```python
from build123d import *

# Parameters (mm, degrees)
F0_W         = 50.8
F0_H         = 50.8
F1_DEPTH     = 50.8
F2_R         = 2.2225
F3_DEPTH     = 3.175
F5_R         = 5.08
F6_T1_DEPTH  = 40.64
F6_T3_DEPTH  = 58.42
F6_T6_ANGLE  = 90
F6_T10_DEPTH = 26.67
F6_T16_DEPTH = 26.67
F6_T22_DEPTH = 26.67
F6_T27_ANGLE = 90
F6_T31_DEPTH = 26.67
F6_T38_DEPTH = 26.67
F6_T44_DEPTH = 26.67
F6_T48_ANGLE = 90
F6_T50_ANGLE = 90
F7_R         = 3.175
F8_DEPTH     = 15.24
F7_W         = 1.27
F7_H         = 6.35
F9_DEPTH     = 8.255


# Not quite as in the source:
# - a fillet or chamfer that OpenCascade refuses, or shapes differently, is made with other operations: its cross-section is extruded or revolved along the edge and cut away or added
# - a feature of the source that left no trace in its solid (it failed there, or was rolled back) is left out


with BuildPart() as f1:
    # F0 (on Top) → F1 (new body)
    with BuildSketch(Plane.XY):
        with Locations((-4.6946440548, -2.4632510453)):
            Rectangle(F0_W, F0_H)
    extrude(amount=F1_DEPTH)

    # F2 (on face) → F3 (join)
    with BuildSketch(Plane(origin=(0, 22.9367489547, 0), x_dir=(-1, 0, 0), z_dir=(0, 1, 0))):
        Polygon((-0.3853559452, 62.23), (-0.3853559452, 53.34), (9.7746440548, 53.34), (9.7746440548, 62.23), (8.5046440548, 63.5), (0.8846440548, 63.5), align=None)
        with Locations((4.6946440548, 58.42)):
            Circle(F2_R, mode=Mode.SUBTRACT)
        Polygon((-0.3853559452, 53.34), (-1.6553559452, 50.8), (11.0446440548, 50.8), (9.7746440548, 53.34), align=None)
    extrude(amount=-F3_DEPTH)

    # F5
    f5_edges = [f1.edges().sort_by_distance(p)[0] for p in [
        (-30.094644, -2.463251, 50.8),
        (20.705356, -2.463251, 50.8),
    ]]
    fillet(f5_edges, radius=F5_R)

    # F6: fillet of radius 5.08 on 11 edges, made by hand

    # F6_s2 → F6_t1 (cut)
    with BuildSketch(Plane.YZ.offset(-25.0146440548)):
        with BuildLine():
            ThreePointArc((-27.8632510453, 45.72), (-26.3753534938, 49.3121024484), (-22.7832510453, 50.8))
            Line((-22.7832510453, 50.8), (-27.8632510453, 50.8))
            Line((-27.8632510453, 50.8), (-27.8632510453, 45.72))
        make_face()
    extrude(amount=F6_T1_DEPTH, mode=Mode.SUBTRACT)

    # F6_s4 → F6_t3 (cut)
    with BuildSketch(Plane.XY.offset(-12.7)):
        with BuildLine():
            ThreePointArc((-30.0946440548, 17.8567489547), (-28.6067465032, 21.4488514031), (-25.0146440548, 22.9367489547))
            Line((-25.0146440548, 22.9367489547), (-30.0946440548, 22.9367489547))
            Line((-30.0946440548, 22.9367489547), (-30.0946440548, 17.8567489547))
        make_face()
        with BuildLine():
            ThreePointArc((-30.0946440548, -22.7832510453), (-28.6067465032, -26.3753534938), (-25.0146440548, -27.8632510453))
            Line((-25.0146440548, -27.8632510453), (-30.0946440548, -27.8632510453))
            Line((-30.0946440548, -27.8632510453), (-30.0946440548, -22.7832510453))
        make_face()
        with BuildLine():
            ThreePointArc((15.6253559452, 22.9367489547), (19.2174583937, 21.4488514031), (20.7053559452, 17.8567489547))
            Line((20.7053559452, 17.8567489547), (20.7053559452, 22.9367489547))
            Line((20.7053559452, 22.9367489547), (15.6253559452, 22.9367489547))
        make_face()
        with BuildLine():
            ThreePointArc((15.6253559452, -27.8632510453), (19.2174583937, -26.3753534938), (20.7053559452, -22.7832510453))
            Line((20.7053559452, -22.7832510453), (20.7053559452, -27.8632510453))
            Line((20.7053559452, -27.8632510453), (15.6253559452, -27.8632510453))
        make_face()
    extrude(amount=F6_T3_DEPTH, mode=Mode.SUBTRACT)

    # F6_s5 → F6_t6 (revolve, cut)
    with BuildSketch(Plane.YZ.offset(15.6253559452)):
        with BuildLine():
            ThreePointArc((22.9367489547, 45.72), (21.4488514031, 49.3121024484), (17.8567489547, 50.8))
            Line((17.8567489547, 50.8), (22.9367489547, 50.8))
            Line((22.9367489547, 50.8), (22.9367489547, 45.72))
        make_face()
    revolve(axis=Axis((15.6253559452, 22.9367489547, 45.72), (0, 1, 0)), revolution_arc=F6_T6_ANGLE, mode=Mode.SUBTRACT)


with BuildPart() as f6_tool8:
    # F6_s9 → F6_t10 (new body)
    with BuildSketch(Plane.YZ.offset(15.6253559452)):
        with BuildLine():
            ThreePointArc((22.9367489547, 45.72), (21.4488514031, 49.3121024484), (17.8567489547, 50.8))
            Line((17.8567489547, 50.8), (22.9367489547, 50.8))
            Line((22.9367489547, 50.8), (22.9367489547, 45.72))
        make_face()
    extrude(amount=-F6_T10_DEPTH)

    split(bisect_by=Plane.XZ.offset(-19.7617489547), keep=Keep.BOTTOM)

    split(bisect_by=Plane(origin=(21.6442847562, 0, 10.8221423781), x_dir=(0, 1, 0), z_dir=(0.894427191, 0, 0.4472135955)), keep=Keep.TOP)


with BuildPart() as f1_1:
    add(f1.part)

    # F6_t7: cut F6_tool8
    add(f6_tool8.part, mode=Mode.SUBTRACT)


with BuildPart() as f6_tool14:
    # F6_s15 → F6_t16 (new body)
    with BuildSketch(Plane.YZ.offset(15.6253559452)):
        with BuildLine():
            ThreePointArc((22.9367489547, 45.72), (21.4488514031, 49.3121024484), (17.8567489547, 50.8))
            Line((17.8567489547, 50.8), (22.9367489547, 50.8))
            Line((22.9367489547, 50.8), (22.9367489547, 45.72))
        make_face()
    extrude(amount=-F6_T16_DEPTH)

    split(bisect_by=Plane.XZ.offset(-19.7617489547), keep=Keep.TOP)

    split(bisect_by=Plane(origin=(21.6442847562, 0, 10.8221423781), x_dir=(0, 1, 0), z_dir=(0.894427191, 0, 0.4472135955)), keep=Keep.TOP)


with BuildPart() as f1_2:
    add(f1_1.part)

    # F6_t13: cut F6_tool14
    add(f6_tool14.part, mode=Mode.SUBTRACT)


with BuildPart() as f6_tool20:
    # F6_s21 → F6_t22 (new body)
    with BuildSketch(Plane.YZ.offset(15.6253559452)):
        with BuildLine():
            ThreePointArc((22.9367489547, 45.72), (21.4488514031, 49.3121024484), (17.8567489547, 50.8))
            Line((17.8567489547, 50.8), (22.9367489547, 50.8))
            Line((22.9367489547, 50.8), (22.9367489547, 45.72))
        make_face()
    extrude(amount=-F6_T22_DEPTH)

    split(bisect_by=Plane(origin=(-29.1557152438, 0, 14.5778576219), x_dir=(0, 1, 0), z_dir=(0.894427191, 0, -0.4472135955)), keep=Keep.TOP)

    split(bisect_by=Plane.XZ.offset(-19.7617489547), keep=Keep.TOP)

    split(bisect_by=Plane(origin=(21.6442847562, 0, 10.8221423781), x_dir=(0, 1, 0), z_dir=(-0.894427191, 0, -0.4472135955)), keep=Keep.TOP)


with BuildPart() as f1_3:
    add(f1_2.part)

    # F6_t19: cut F6_tool20
    add(f6_tool20.part, mode=Mode.SUBTRACT)

    # F6_s26 → F6_t27 (revolve, cut)
    with BuildSketch(Plane.XY.offset(45.72)):
        with BuildLine():
            ThreePointArc((-25.0146440548, 22.9367489547), (-28.6067465032, 21.4488514031), (-30.0946440548, 17.8567489547))
            Line((-30.0946440548, 17.8567489547), (-30.0946440548, 22.9367489547))
            Line((-30.0946440548, 22.9367489547), (-25.0146440548, 22.9367489547))
        make_face()
    revolve(axis=Axis((-25.0146440548, 22.9367489547, 45.72), (0, 1, 0)), revolution_arc=F6_T27_ANGLE, mode=Mode.SUBTRACT)


with BuildPart() as f6_tool29:
    # F6_s30 → F6_t31 (new body)
    with BuildSketch(Plane.YZ.offset(1.6553559452)):
        with BuildLine():
            ThreePointArc((22.9367489547, 45.72), (21.4488514031, 49.3121024484), (17.8567489547, 50.8))
            Line((17.8567489547, 50.8), (22.9367489547, 50.8))
            Line((22.9367489547, 50.8), (22.9367489547, 45.72))
        make_face()
    extrude(amount=-F6_T31_DEPTH)

    split(bisect_by=Plane(origin=(-29.1557152438, 0, 14.5778576219), x_dir=(0, 1, 0), z_dir=(0.894427191, 0, -0.4472135955)), keep=Keep.TOP)

    split(bisect_by=Plane.XZ.offset(-19.7617489547), keep=Keep.TOP)

    split(bisect_by=Plane(origin=(21.6442847562, 0, 10.8221423781), x_dir=(0, 1, 0), z_dir=(-0.894427191, 0, -0.4472135955)), keep=Keep.TOP)


with BuildPart() as f1_4:
    add(f1_3.part)

    # F6_t28: cut F6_tool29
    add(f6_tool29.part, mode=Mode.SUBTRACT)


with BuildPart() as f6_tool36:
    # F6_s37 → F6_t38 (new body)
    with BuildSketch(Plane.YZ.offset(1.6553559452)):
        with BuildLine():
            ThreePointArc((22.9367489547, 45.72), (21.4488514031, 49.3121024484), (17.8567489547, 50.8))
            Line((17.8567489547, 50.8), (22.9367489547, 50.8))
            Line((22.9367489547, 50.8), (22.9367489547, 45.72))
        make_face()
    extrude(amount=-F6_T38_DEPTH)

    split(bisect_by=Plane(origin=(-29.1557152438, 0, 14.5778576219), x_dir=(0, 1, 0), z_dir=(-0.894427191, 0, 0.4472135955)), keep=Keep.TOP)

    split(bisect_by=Plane.XZ.offset(-19.7617489547), keep=Keep.BOTTOM)


with BuildPart() as f1_5:
    add(f1_4.part)

    # F6_t35: cut F6_tool36
    add(f6_tool36.part, mode=Mode.SUBTRACT)


with BuildPart() as f6_tool42:
    # F6_s43 → F6_t44 (new body)
    with BuildSketch(Plane.YZ.offset(1.6553559452)):
        with BuildLine():
            ThreePointArc((22.9367489547, 45.72), (21.4488514031, 49.3121024484), (17.8567489547, 50.8))
            Line((17.8567489547, 50.8), (22.9367489547, 50.8))
            Line((22.9367489547, 50.8), (22.9367489547, 45.72))
        make_face()
    extrude(amount=-F6_T44_DEPTH)

    split(bisect_by=Plane(origin=(-29.1557152438, 0, 14.5778576219), x_dir=(0, 1, 0), z_dir=(-0.894427191, 0, 0.4472135955)), keep=Keep.TOP)

    split(bisect_by=Plane.XZ.offset(-19.7617489547), keep=Keep.TOP)


with BuildPart() as f1_6:
    add(f1_5.part)

    # F6_t41: cut F6_tool42
    add(f6_tool42.part, mode=Mode.SUBTRACT)

    # F6_s47 → F6_t48 (revolve, cut)
    with BuildSketch(Plane.XY.offset(45.72)):
        with BuildLine():
            ThreePointArc((-30.0946440548, -22.7832510453), (-28.6067465032, -26.3753534938), (-25.0146440548, -27.8632510453))
            Line((-25.0146440548, -27.8632510453), (-30.0946440548, -27.8632510453))
            Line((-30.0946440548, -27.8632510453), (-30.0946440548, -22.7832510453))
        make_face()
    revolve(axis=Axis((-25.0146440548, -27.8632510453, 45.72), (0, 1, 0)), revolution_arc=F6_T48_ANGLE, mode=Mode.SUBTRACT)

    # F6_s49 → F6_t50 (revolve, cut)
    with BuildSketch(Plane.YZ.offset(15.6253559452)):
        with BuildLine():
            ThreePointArc((-27.8632510453, 45.72), (-26.3753534938, 49.3121024484), (-22.7832510453, 50.8))
            Line((-22.7832510453, 50.8), (-27.8632510453, 50.8))
            Line((-27.8632510453, 50.8), (-27.8632510453, 45.72))
        make_face()
    revolve(axis=Axis((15.6253559452, -27.8632510453, 45.72), (0, 1, 0)), revolution_arc=F6_T50_ANGLE, mode=Mode.SUBTRACT)

    # F7 (on face) → F8 (join)
    with BuildSketch(Plane(origin=(0, 0, 0), x_dir=(1, 0, 0), z_dir=(0, 0, -1))):
        with Locations((-20.5696440548, 11.9882510453)):
            Circle(F7_R)
        with Locations((11.1803559452, 11.9882510453)):
            Circle(F7_R)
    extrude(amount=F8_DEPTH)

    # F7 (on face) → F9 (join)
    with BuildSketch(Plane(origin=(0, 0, 0), x_dir=(1, 0, 0), z_dir=(0, 0, -1))):
        with Locations((-7.8696440548, -7.0617489547)):
            Rectangle(F7_W, F7_H)
        with Locations((-1.5196440548, -7.0617489547)):
            Rectangle(F7_W, F7_H)
    extrude(amount=F9_DEPTH)


solid = f1_6.part
```
Geometry check sheet. Reference: the model listing, model coordinates, mm. A direction names the side the tool comes from. Round coordinates to 2 decimals unless told otherwise and drop trailing zeros. Loops run counter-clockwise (first coordinate to the right, second up) from the corner with the lowest first, then second, coordinate; pieces in that order, holes last. Notation, with made-up numbers: (-26.75, 27.25) -> (10.25, 27.25) arc R20 ccw to (10.25, 44.25) -> close; hole circle Ø4 at (-27.5, 8.5). An arc over 180 degrees is marked (long way). Use a Markdown table: item, result.
(1) Sectioned sample at A-A (z = 58.42). Enter the section's corners in (x, y), then the cut area to 3 significant figures.
Calculated:
| item | result |
|---|---|
| outline | (-9.77, 19.76) -> (-6.92, 19.76) -> (-6.92, 22.94) -> (-9.77, 22.94) -> close; (-2.47, 19.76) -> (0.39, 19.76) -> (0.39, 22.94) -> (-2.47, 22.94) -> close |
| area | 18.1 mm² |
(2) Sectioned sample at B-B (x = 6.5). Enter the section's corners in (y, z).
Calculated:
| item | result |
|---|---|
| outline | (-27.86, 0) -> (22.94, 0) -> (22.94, 45.72) arc R5.08 ccw to (17.86, 50.8) -> (-22.78, 50.8) arc R5.08 ccw to (-27.86, 45.72) -> close |
(3) Sectioned sample at D-D (x = -5). Enter the section's corners in (y, z).
Calculated:
| item | result |
|---|---|
| outline | (-27.86, 0) -> (22.94, 0) -> (22.94, 56.22) -> (19.76, 56.22) -> (19.76, 50.43) arc R5.08 ccw to (17.86, 50.8) -> (-22.78, 50.8) arc R5.08 ccw to (-27.86, 45.72) -> close; (19.76, 60.62) -> (22.94, 60.62) -> (22.94, 63.5) -> (19.76, 63.5) -> close |
(4) Set-up check for faces 4 (the flat face through (-0.885, 7, -4)), 5 (the flat face through (0.385, 21, 58)), 6 (the flat face through (-9.775, 21, 58)), 7 (the cylindrical face through (-17.54, -12.94, -7.51)): record each of +Z, -Z, +X, -X, +Y, -Y from which the full face is reachable in a straight line by a thin tool's end or side.
Calculated:
| item | result |
|---|---|
| face 4 | -Z, +X, +Y, -Y |
| face 5 | +Z, +X, +Y, -Y |
| face 6 | +Z, -X, +Y, -Y |
| face 7 | -Z |
(5) Go/stop test with flat-tipped pins: P1, Ø7, axis at y = 7.5, z = -4, coming from the -X side; P2, Ø1.4, axis at x = -8, y = 7, coming from the -Z side (3 decimals); P3, Ø5, axis at x = -3, y = -17, coming from the +Z side. Record where each tip stops, or that it passes through.
Calculated:
| item | result |
|---|---|
| P1 | x = -8.5 |
| P2 | z = -8.255 |
| P3 | z = 50.8 |
(6) Sectioned sample at C-C (y = 13). Enter the section's corners in (x, z), then the cut area to 3 significant figures.
Calculated:
| item | result |
|---|---|
| outline | (-30.09, 0) -> (20.71, 0) -> (20.71, 45.72) arc R5.08 ccw to (15.63, 50.8) -> (-25.01, 50.8) arc R5.08 ccw to (-30.09, 45.72) -> close |
| area | 2,570 mm² |
(7) Mould release check, pull along X, two halves, no side actions. Record for faces 1 (the flat face through (1.417, 21.68, 51.277)), 2 (the flat face through (-7.235, 7, -4)), 3 (the flat face through (-8.505, 7, -4)): released by +X, released by -X, zero draft, split by the parting line, or undercut.
Calculated:
| item | result |
|---|---|
| face 1 | released by +X |
| face 2 | undercut |
| face 3 | released by -X |
(8) Scan lines: probe 1 along Z at (x, y) = (-20, -5.5); probe 2 along Y at (x, z) = (-5.5, 56); probe 3 along Z at (x, y) = (-19.5, -11.5). Record each from-to range of solid material in increasing order.
Calculated:
| item | result |
|---|---|
| probe 1 | 0 to 50.8 |
| probe 2 | 19.76 to 22.94 |
| probe 3 | -15.24 to 50.8 |
